Check sheet for the modelled part. Datum: model origin and axes. Units: mm. Face numbers are marked on the shaded views. A direction names the side the tool comes from. Give positions to 0.01 mm unless a question says otherwise; leave off trailing zeros. Order: outer loops, then holes, each group sorted by start corner. A loop starts at its lowest first (then second) coordinate and runs counter-clockwise, first axis right, second up.
Item 1: Access from +Z, -Z, +X, -X, +Y, -Y to the whole of each face (thin tool, end or side, straight path). Record for the marked faces 1, 2 and 3.
Item 2: Sectioned sample at A-A on z = -40. Record the boundary of the cut face in (x, y).
Item 3: Sectioned sample at B-B on x = 0. Record the boundary of the cut face in (y, z), and give its area (3 significant figures).
Item 4: Sectioned sample at C-C on z = 0. Record the boundary of the cut face in (x, y).
Item 5: Sectioned sample at D-D on y = 9. Count the separate pieces of the cut face and the enclosed holes in it, and give its area (3 significant figures).
Item 6: Gauge pin test, flat ends, axial feed: P1, Ø5.5, axis at y = 8, z = 40, coming from the +X side; P2, Ø10, axis at x = -7.5, z = -18, coming from the +Y side; P3, Ø13, axis at x = -15.1, z = 0, coming from the +Y side; P4, Ø7.5, axis at y = 7.5, z = 42, coming from the -X side. Record the tip position at first contact, or that the pin passes through.
Item 7: Release check for a two-part mould opening along Z. For the marked faces 4, 5 and 6 record: released by +Z, released by -Z, zero draft, split by the parting line, or undercut.
Item 8: Material ranges on line 1 along Z through (x, y) = (0, 9.75); line 2 along Z through (x, y) = (16, 4); line 3 along X through (y, z) = (3.75, -17), recorded low to high.
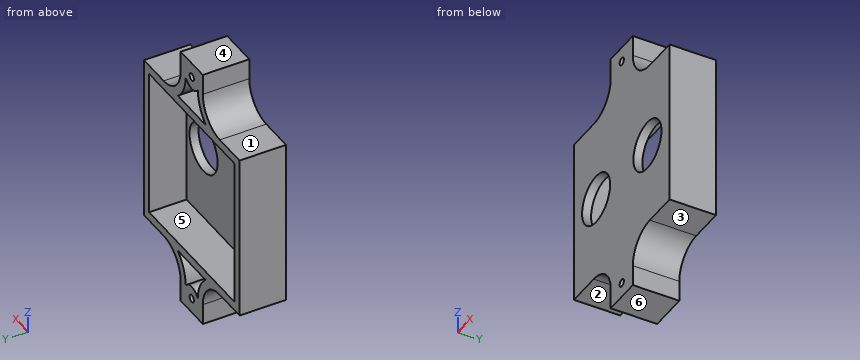
from build123d import *

# Parameters (mm, degrees)
F0_W        = 56.2
F0_H        = 56
F0_W_2      = 50.2
F0_H_2      = 50
F0_R        = 8.25
F1_DEPTH    = 3
F2_DEPTH    = 12.5
F3_W        = 13
F3_H        = 17
F3_R        = 1.25
F4_DEPTH    = 15.5
F5_R        = 10
F6_T        = 3
F6_T3_DEPTH = 56.2
F6_T5_DEPTH = 56
F6_T7_DEPTH = 18.5


# Not quite as in the source:
# - a shell that OpenCascade refuses in one call is made with other operations: the cavity is built on its own and cut out


with BuildPart() as f1:
    # F0 (on Front) → F1 (new body)
    with BuildSketch(Plane.XZ):
        Rectangle(F0_W, F0_H)
        Rectangle(F0_W_2, F0_H_2, mode=Mode.SUBTRACT)
        Rectangle(F0_W_2, F0_H_2)
        with Locations((-15.1, 0)):
            Circle(F0_R, mode=Mode.SUBTRACT)
        with Locations((15.1, 0)):
            Circle(F0_R, mode=Mode.SUBTRACT)
    extrude(amount=F1_DEPTH)

    # F0 (on Front) → F2 (join)
    with BuildSketch(Plane.XZ):
        Rectangle(F0_W, F0_H)
        Rectangle(F0_W_2, F0_H_2, mode=Mode.SUBTRACT)
    extrude(amount=-F2_DEPTH)

    # F3 (on face) → F4 (join, through all)
    with BuildSketch(Plane.XZ.offset(3)):
        with Locations((0, 36.5)):
            Rectangle(F3_W, F3_H)
        with Locations((0, 40)):
            Circle(F3_R, mode=Mode.SUBTRACT)
        with Locations((0, -36.5)):
            Rectangle(F3_W, F3_H)
        with Locations((0, -40)):
            Circle(F3_R, mode=Mode.SUBTRACT)
    extrude(amount=-F4_DEPTH)

    # F5
    f5_edges = [f1.edges().sort_by_distance(p)[0] for p in [
        (6.5, 4.75, -28),
        (-6.5, 4.75, -28),
        (-6.5, 4.75, 28),
        (6.5, 4.75, 28),
    ]]
    fillet(f5_edges, radius=F5_R)

    # F6: shell of thickness 3, made by hand


with BuildPart() as f6_core1:
    # F6_t2: copy of F1
    add(f1.part)

    # the walls: a layer under each face that stays
    f6_faces = [f6_core1.faces().sort_by_distance(p)[0] for p in [
        (0, -3, 0),
        (22.3, 4.75, 28),
        (9.4289321881, 4.75, 30.9289321881),
        (28.1, 4.75, 0),
        (6.5, 4.75, 41.5),
        (22.3, 4.75, -28),
        (0, 4.75, 45),
        (9.4289321881, 4.75, -30.9289321881),
        (-6.5, 4.75, 41.5),
        (6.5, 4.75, -41.5),
        (-9.4289321881, 4.75, 30.9289321881),
        (0, 4.75, -45),
        (-22.3, 4.75, 28),
        (-6.5, 4.75, -41.5),
        (-28.1, 4.75, 0),
        (-9.4289321881, 4.75, -30.9289321881),
        (-22.3, 4.75, -28),
        (-23.35, -1.5, 0),
        (6.85, -1.5, 0),
        (-1.25, 4.75, 40),
        (-1.25, 4.75, -40),
        (0, 0, 0),
        (0, 6.25, 25),
        (25.1, 6.25, 0),
        (0, 6.25, -25),
        (-25.1, 6.25, 0),
    ]]
    thicken(f6_faces, amount=-F6_T, mode=Mode.SUBTRACT)

    # F6_s4 → F6_t3 (cut)
    with BuildSketch(Plane.YZ.offset(-28.1)):
        Polygon((0.03, 24.97), (-3, 25), (-3, 28), (0, 28), align=None)
        Polygon((0.03, -24.97), (-3, -25), (-3, -28), (0, -28), align=None)
    extrude(amount=F6_T3_DEPTH, mode=Mode.SUBTRACT)

    # F6_s6 → F6_t5 (cut)
    with BuildSketch(Plane.XY.offset(-28)):
        Polygon((25.07, 0.03), (25.1, -3), (28.1, -3), (28.1, 0), align=None)
        Polygon((-25.07, 0.03), (-25.1, -3), (-28.1, -3), (-28.1, 0), align=None)
    extrude(amount=F6_T5_DEPTH, mode=Mode.SUBTRACT)

    # F6_s8 → F6_t7 (cut)
    with BuildSketch(Plane.XZ.offset(-15.5)):
        Polygon((-25.07, 24.97), (-25.1, 28), (-28.1, 28), (-28.1, 25), align=None)
        Polygon((25.07, 24.97), (25.1, 28), (28.1, 28), (28.1, 25), align=None)
        Polygon((25.07, -24.97), (28.1, -25), (28.1, -28), (25.1, -28), align=None)
        Polygon((-25.07, -24.97), (-25.1, -28), (-28.1, -28), (-28.1, -25), align=None)
    extrude(amount=F6_T7_DEPTH, mode=Mode.SUBTRACT)


with BuildPart() as f1_1:
    add(f1.part)

    # what is left inside the walls is the cavity
    f6_cavity = [f6_core1.part.solids().sort_by_distance(p)[0] for p in [
        (0, 8.333333, 28.03),
        (0, 8.333333, -28.03),
    ]]
    add(f6_cavity, mode=Mode.SUBTRACT)


solid = f1_1.part
Report:
1. face 1: +Z, -X, +Y, -Y
1. face 2: -Z, -X, +Y, -Y
1. face 3: -Z, +X, +Y, -Y
2. outline: (-6.5, -3) - (-1.25, -3) - (-1.25, 12.5) - (-6.5, 12.5) - close; (1.25, -3) - (6.5, -3) - (6.5, 12.5) - (1.25, 12.5) - close
3. outline: (-3, -45) - (12.5, -45) - (12.5, -41.25) - (-3, -41.25) - close; (-3, -38.75) - (12.5, -38.75) - (12.5, -35.75) - (0, -35.75) - (0, -28) - (12.5, -28) - (12.5, -25) - (0, -25) - (0, 25) - (12.5, 25) - (12.5, 28) - (0, 28) - (0, 35.75) - (12.5, 35.75) - (12.5, 38.75) - (-3, 38.75) - close; (-3, 41.25) - (12.5, 41.25) - (12.5, 45) - (-3, 45) - close
3. area: 499 mm2
4. outline: (-28.1, -3) - (-23.35, -3) - (-23.35, 0) - (-25.1, 0) - (-25.1, 12.5) - (-28.1, 12.5) - close; (-6.85, -3) - (6.85, -3) - (6.85, 0) - (-6.85, 0) - close; (23.35, -3) - (28.1, -3) - (28.1, 12.5) - (25.1, 12.5) - (25.1, 0) - (23.35, 0) - close
5. separate pieces: 1
5. enclosed holes: 5
5. area: 982 mm2
6. P1: stops at x = 6.53
6. P2: stops at y = 0
6. P3: passes through
6. P4: stops at x = -6.5
7. face 4: released by +Z
7. face 5: undercut
7. face 6: released by -Z
8. line 1: z = -45 to -41.25, -38.75 to -35.75, -28 to -25, 25 to 28, 35.75 to 38.75, 41.25 to 45
8. line 2: z = -28.01 to -25, 25 to 28.01
8. line 3: x = -28.1 to -25.1, 25.1 to 28.1
